Source: three-view drawing plus pictorial views. Frame: mm from the lowest corner of the part. A direction names the side the tool comes from. Round coordinates to 2 decimals unless told otherwise and drop trailing zeros. Write each loop counter-clockwise with the first axis right and the second up, starting at its lowest first coordinate (ties: lowest second). Pieces come first, ordered by that corner, then holes. Notation, with made-up numbers: (7.5, 79.5) - (13.5, 79.5) arc R19 ccw to (13.5, 105.5) - close; hole circle Ø8 at (66.25, 27.5). An arc over 180 degrees is marked (long way). Write each question's results on one line, items separated by ' | '.
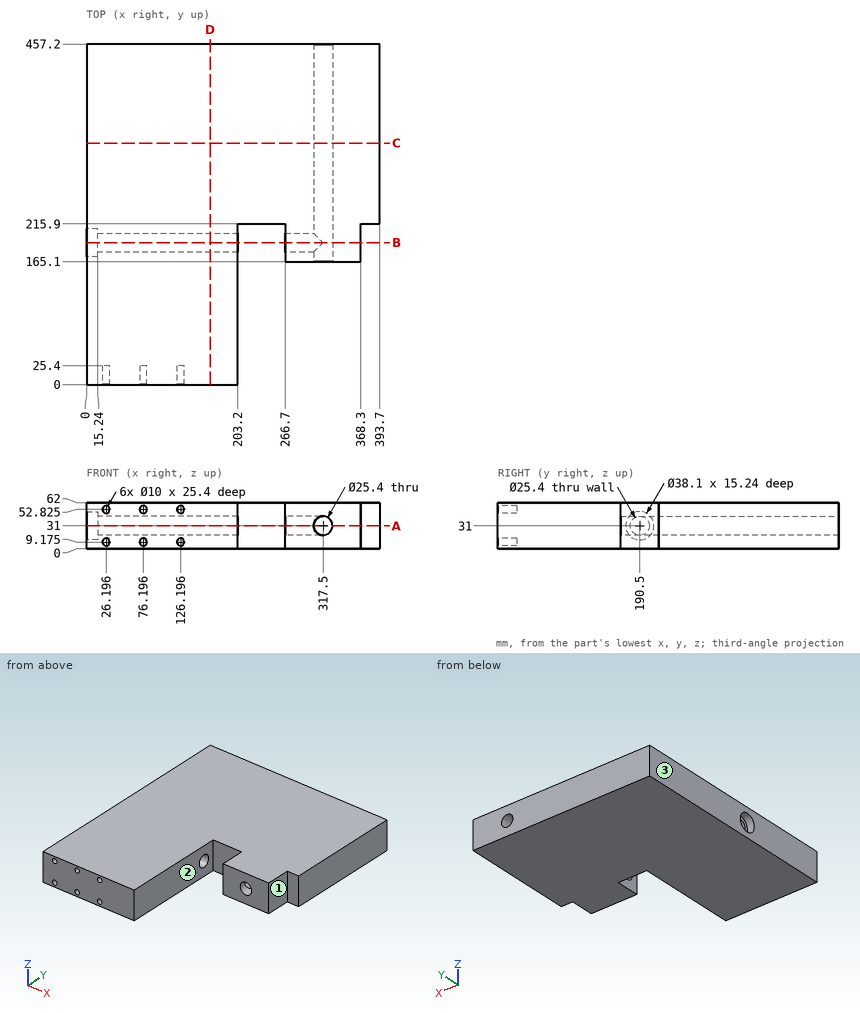
Q1. Section query A-A, the plane z = 31. Return loops of the section in (x, y), plus the area to 3 significant figures.
Answer block:
outline: (0, 0) - (203.2, 0) - (203.2, 177.8) - (15.24, 177.8) - (15.24, 171.45) - (0, 171.45) - close; (0, 209.55) - (15.24, 209.55) - (15.24, 203.2) - (203.2, 203.2) - (203.2, 215.9) - (266.7, 215.9) - (266.7, 203.2) - (304.8, 203.2) - (304.8, 457.2) - (0, 457.2) - close; (266.7, 165.1) - (304.8, 165.1) - (304.8, 177.8) - (266.7, 177.8) - close; (330.2, 165.1) - (368.3, 165.1) - (368.3, 215.9) - (393.7, 215.9) - (393.7, 457.2) - (330.2, 457.2) - close | area: 130,000 mm2
Q2. Section query B-B, the plane y = 190.5. Return loops of the section in (x, z), plus the area to 3 significant figures.
Answer block:
outline: (0, 0) - (203.2, 0) - (203.2, 18.3) - (15.24, 18.3) - (15.24, 11.95) - (0, 11.95) - close; (0, 50.05) - (15.24, 50.05) - (15.24, 43.7) - (203.2, 43.7) - (203.2, 62) - (0, 62) - close; (266.7, 0) - (368.3, 0) - (368.3, 62) - (266.7, 62) - (266.7, 43.7) - (317.5, 43.7) arc R12.7 cw to (317.5, 18.3) - (266.7, 18.3) - close | area: 12,000 mm2
Q3. Section query D-D, the plane x = 166. Return loops of the section in (y, z).
Answer block:
outline: (0, 0) - (457.2, 0) - (457.2, 62) - (0, 62) - close; hole circle Ø25.4 at (190.5, 31)
Q4. Ray query, line 1 along X through (y, z) = (226, 31); line 2 along X through (y, z) = (209.5, 52.5); line 3 along Y through (x, z) = (93, 31). Return the intervals inside material, ascending.
Answer block:
line 1: 0 to 304.8, 330.2 to 393.7 | line 2: 0 to 203.2, 266.7 to 368.3 | line 3: 0 to 177.8, 203.2 to 457.2
Q5. Section query C-C, the plane y = 324. Return loops of the section in (x, z), plus the area to 3 significant figures.
Answer block:
outline: (0, 0) - (393.7, 0) - (393.7, 62) - (0, 62) - close; hole circle Ø25.4 at (317.5, 31) | area: 23,900 mm2
Q6. Pin query (flat end, axial travel): pin 1 (15 mm diameter, centred on y = 190.5, z = 31, fed in from -X); pin 2 (3 mm diameter, centred on x = 127, z = 55, fed in from -Y); pin 3 (2 mm diameter, centred on y = 145, z = 36, fed in from +X). Return the tip coordinate at first contact, or that it passes through.
Answer block:
pin 1: x = 327.75 | pin 2: y = 25.4 | pin 3: x = 203.2
Q7. Access query for the marked faces 1, 2 and 3. Directions: +Z, -Z, +X, -X, +Y, -Y. A direction counts if a zero-diameter tool reaches every point of the face in a straight line with its end or side. Return the directions, or none.
Answer block:
face 1: +Z, -Z, +X, -Y | face 2: +Z, -Z, -Y | face 3: +Z, -Z, -X, +Y, -Y
